Build history of the part. All positions in model axes, mm. A direction names the side the tool comes from. Round coordinates to 2 decimals unless told otherwise and drop trailing zeros. Order: outer loops, then holes, each group sorted by start corner. A loop starts at its lowest first (then second) coordinate and runs counter-clockwise, first axis right, second up. Notation, with made-up numbers: M 23.5,52.5 L 59.5,52.5 A6 cw 59.5,56.5 Z; hole C 63.5,-3.75 d10. An arc over 180 degrees is marked long. One line per item, written item: value. Start each with the question number.
Item 1: Band-saw the part on A-A, the plane z = 0. Write the cut outline in (x, y).
Item 2: Probe L1, parallel to Z at x = 22, y = -4.25; L2, parallel to X at y = -11, z = -5; L3, parallel to Z at x = -60, y = -13.25. List the from-to ranges inside material, lowest first.
Item 3: Two-plate mould, pull along X, no slides. Class faces 5 (the flat face through (-42, -6, -12.5)), 6 (the flat face through (-77.5, -7, 0)), 7 (the flat face through (-61, -7, -42.5)): +X half, -X half, draft (parallel to the pull), parting line (faces both ways), or undercut.
Item 4: Band-saw the part on B-B, the plane y = -10.25. Write the cut outline in (x, z), then the cut area to 3 significant figures.
Item 5: Tool access for faces 1 (the cylindrical face through (-29.2, -14.4, -18.8)), 2 (the flat face through (-72, -7, -12.5)), 3 (the flat face through (32, 0, -3)), 4 (the flat face through (-29.049, -7.423, -19.794)): list every direction of +Z, -Z, +X, -X, +Y, -Y with a clear straight run to the whole face (end or side of a thin tool).
Item 6: Pin check, flat tips, straight feed: pin 1 (5.5 mm diameter, centred on x = -44.5, y = -4.5, fed in from -Z); pin 2 (8 mm diameter, centred on x = 98.5, y = -11, fed in from -Z); pin 3 (2 mm diameter, centred on y = -13, z = -6.5, fed in from +X). Stop position of each tip, or through.
Item 7: Band-saw the part on C-C, the plane x = -13.5. Write the cut outline in (y, z), then the cut area to 3 significant figures.
```python
from build123d import *

# Parameters (mm, degrees)
F0_R     = 17.5
F0_W     = 8
F0_H     = 15
F0_W_2   = 10
F0_H_2   = 30
F1_DEPTH = 15
F2_R     = 2


with BuildPart() as f1:
    # F0 (on Front) → F1 (new body)
    with BuildSketch(Plane.XZ):
        Polygon((77.5, 12.5), (-77.5, 12.5), (-77.5, -12.5), (-65.925811, -12.5), (-55.925811, -12.5), (-52.329316, -12.5), (-44.329316, -12.5), (-39.5, -12.5), (-32.5, -12.5), (-25.5, -12.5), (77.5, -12.5), align=None)
        with BuildLine():
            ThreePointArc((77.5, -12.5), (145.191742, 0), (77.5, 12.5))
            Line((77.5, 12.5), (77.5, -12.5))
        make_face()
        with Locations((110.191742, 0)):
            Circle(F0_R, mode=Mode.SUBTRACT)
        Polygon((-32.5, -26.887495), (-32.5, -12.5), (-39.5, -12.5), align=None)
        Polygon((-32.5, -26.887495), (-25.5, -12.5), (-32.5, -12.5), align=None)
        with Locations((-48.329316, -20)):
            Rectangle(F0_W, F0_H)
        with Locations((-60.925811, -27.5)):
            Rectangle(F0_W_2, F0_H_2)
    extrude(amount=F1_DEPTH)

    # F2
    f2_edges = [f1.edges().sort_by_distance(p)[0] for p in [
        (0, -15, 12.5),
        (-77.5, -15, 0),
        (-71.712905, -15, -12.5),
        (-65.925811, -15, -27.5),
        (-60.925811, -15, -42.5),
        (-55.925811, -15, -27.5),
        (-54.127563, -15, -12.5),
        (-52.329316, -15, -20),
        (-48.329316, -15, -27.5),
        (-44.329316, -15, -20),
        (-41.914658, -15, -12.5),
        (-36, -15, -19.693747),
        (-29, -15, -19.693747),
        (26, -15, -12.5),
        (145.191742, -15, 0),
        (92.691742, -15, 0),
        (-29, 0, -19.693747),
        (92.691742, 0, 0),
        (0, 0, 12.5),
        (-77.5, 0, 0),
        (-60.925811, 0, -42.5),
        (-55.925811, 0, -27.5),
        (-52.329316, 0, -20),
        (145.191742, 0, 0),
        (-44.329316, 0, -20),
        (-71.712905, 0, -12.5),
    ]]
    fillet(f2_edges, radius=F2_R)


solid = f1.part
```
Output:
1. outline: M -77.5,-13 A2 ccw -75.5,-15 L 90.69,-15 A2 ccw 92.69,-13 L 92.69,-2 A2 ccw 90.69,0 L -75.5,0 A2 ccw -77.5,-2 Z; M 127.69,-13 A2 ccw 129.69,-15 L 143.19,-15 A2 ccw 145.19,-13 L 145.19,-2 A2 ccw 143.19,0 L 129.69,0 A2 ccw 127.69,-2 Z
2. L1: z = -12.5 to 12.5
2. L2: x = -77.5 to 93.42, 126.96 to 144.83
2. L3: z = -42.48 to 12.48
3. face 5: undercut
3. face 6: -X half
3. face 7: draft
4. outline: M -77.5,-12.5 L -65.93,-12.5 L -65.93,-42.5 L -55.93,-42.5 L -55.93,-12.5 L -52.33,-12.5 L -52.33,-27.5 L -44.33,-27.5 L -44.33,-12.5 L -39.5,-12.5 L -32.5,-26.89 L -25.5,-12.5 L 77.5,-12.5 A35 ccw long 77.5,12.5 L -77.5,12.5 Z; hole C 110.19,0 d35
4. area: 7,240 mm²
5. face 1: -Z, -Y
5. face 2: -Z, -X, +Y, -Y
5. face 3: +Z, -Z, +X, -X, +Y
5. face 4: -Z, +Y, -Y
6. pin 1: stops at z = -27.5
6. pin 2: stops at z = -34.14
6. pin 3: stops at x = 144.76
7. outline: M -15,-10.5 A2 ccw -13,-12.5 L 0,-12.5 L 0,10.5 A2 ccw -2,12.5 L -13,12.5 A2 ccw -15,10.5 Z
7. area: 372 mm²
